Drawing for the job (mm, zero at the part's lowest x, y, z). A direction names the side the tool comes from. Coordinates: 2 decimals unless noted, no trailing zeros. Write each loop counter-clockwise with the first axis right and the second up, starting at its lowest first coordinate (ties: lowest second). Pieces come first, ordered by that corner, then holes. Notation, with made-up numbers: (22.25, 84.25) - (66.25, 84.25) arc R18 ccw to (66.25, 103.25) - close; hole circle Ø3 at (26.25, -18). An arc over 180 degrees is marked (long way). Write each question's results on one line, items separated by ' | '.
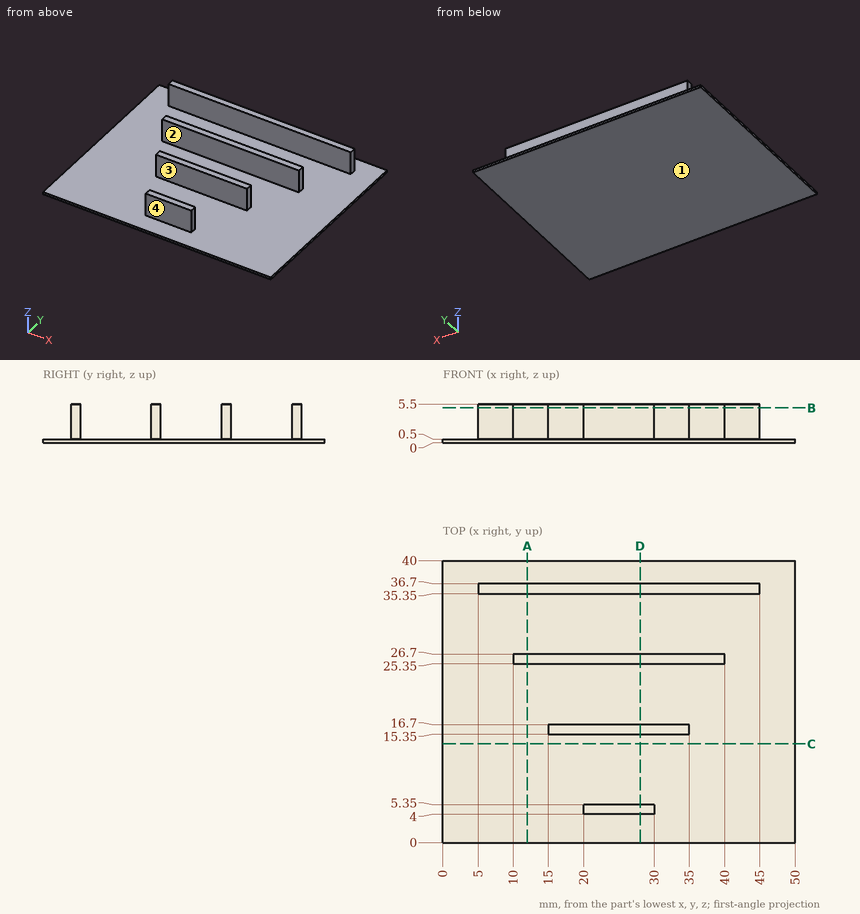
(1) Saw through at B-B on z = 4.95. Write the cut outline in (x, y).
Return value:
outline: (5, 35.35) - (45, 35.35) - (45, 36.7) - (5, 36.7) - close; (10, 25.35) - (40, 25.35) - (40, 26.7) - (10, 26.7) - close; (15, 15.35) - (35, 15.35) - (35, 16.7) - (15, 16.7) - close; (20, 4) - (30, 4) - (30, 5.35) - (20, 5.35) - close
(2) Two-plate mould, pull along Z, no slides. Class the marked faces 1 and 2: released by +Z, released by -Z, zero draft, split by the parting line, or undercut.
Return value:
face 1: released by -Z | face 2: zero draft
(3) 3-axis set-ups, long thin cutter, end or side, ignore diameter. For the marked faces 3 and 4: which of +Z, -Z, +X, -X, +Y, -Y reach the whole face in a straight line?
Return value:
face 3: +Z, +X, -X | face 4: +Z, +X, -X, -Y
(4) Saw through at D-D on x = 28. Write the cut outline in (y, z).
Return value:
outline: (0, 0) - (40, 0) - (40, 0.5) - (36.7, 0.5) - (36.7, 5.5) - (35.35, 5.5) - (35.35, 0.5) - (26.7, 0.5) - (26.7, 5.5) - (25.35, 5.5) - (25.35, 0.5) - (16.7, 0.5) - (16.7, 5.5) - (15.35, 5.5) - (15.35, 0.5) - (5.35, 0.5) - (5.35, 5.5) - (4, 5.5) - (4, 0.5) - (0, 0.5) - close
(5) Wall check: line 1 (Y direction, x = 34, z = 4.5); line 2 (Y direction, x = 24, z = 1.9); line 3 (X direction, y = 5, z = 2.3). Give the ranges that are in metal, low to high. Write a range as from..to.
Return value:
line 1: y = 15.35..16.7, 25.35..26.7, 35.35..36.7 | line 2: y = 4..5.35, 15.35..16.7, 25.35..26.7, 35.35..36.7 | line 3: x = 20..30
(6) Saw through at A-A on x = 12. Write the cut outline in (y, z).
Return value:
outline: (0, 0) - (40, 0) - (40, 0.5) - (36.7, 0.5) - (36.7, 5.5) - (35.35, 5.5) - (35.35, 0.5) - (26.7, 0.5) - (26.7, 5.5) - (25.35, 5.5) - (25.35, 0.5) - (0, 0.5) - close
(7) Flat gauge pins, fed straight in: P1, Ø1, axis at x = 38.5, y = 31.5, coming from the +Z side; P2, Ø0.7, axis at y = 4.5, z = 2, coming from the -X side; P3, Ø2.5, axis at x = 25.5, z = 2.5, coming from the -Y side. Where does each tip first touch, or does it go through?
Return value:
P1: stops at z = 0.5 | P2: stops at x = 20 | P3: stops at y = 4
(8) Saw through at C-C on y = 14. Write the cut outline in (x, z).
Return value:
outline: (0, 0) - (50, 0) - (50, 0.5) - (0, 0.5) - close
